Build history of the part. All positions in model axes, mm. A direction names the side the tool comes from. Give positions to 0.01 mm unless a question says otherwise; leave off trailing zeros. Order: outer loops, then holes, each group sorted by start corner. A loop starts at its lowest first (then second) coordinate and runs counter-clockwise, first axis right, second up. Notation, with made-up numbers: (9.5, -12.5) - (57.5, -12.5) arc R14 cw to (57.5, 12.5) - close; hole circle Ø6 at (61.5, 39.25). An arc over 180 degrees is marked (long way). Write each question's results on one line, items separated by ' | '. Start each with the question number.
from build123d import *

# Parameters (mm, degrees)
F0_W     = 10
F0_H     = 10
F1_DEPTH = 40
F3_D     = 2.5
F3_DEPTH = 10
F3_TIP   = 0.7510757738
F5_D     = 2.5
F5_DEPTH = 10
F5_TIP   = 0.7510757738


with BuildPart() as f1:
    # F0 (on Right) → F1 (new body)
    with BuildSketch(Plane.YZ):
        with Locations((-5, 5)):
            Rectangle(F0_W, F0_H)
    extrude(amount=F1_DEPTH)

    # F3
    with Locations(Plane.YZ.offset(40)):
        with Locations((-5, 5)):
            Hole(F3_D / 2, depth=F3_DEPTH)
            with Locations((0, 0, -(F3_DEPTH + F3_TIP / 2))):  # 118° drill point
                Cone(0, F3_D / 2, F3_TIP, mode=Mode.SUBTRACT)

    # F5
    with Locations(Plane(origin=(0, 0, 0), x_dir=(0, -1, 0), z_dir=(-1, 0, 0))):
        with Locations((5, 5)):
            Hole(F5_D / 2, depth=F5_DEPTH)
            with Locations((0, 0, -(F5_DEPTH + F5_TIP / 2))):  # 118° drill point
                Cone(0, F5_D / 2, F5_TIP, mode=Mode.SUBTRACT)


solid = f1.part
Item 1: Which spindle directions (+Z, -Z, +X, -X, +Y, -Y) get a long thin tool onto all of the face, cutting with end or side? Do faces 1 (the cylindrical face through (34.93, -4.73, 3.78)), 2 (the cylindrical face through (5.07, -5.27, 3.78)), 3 (the flat face through (20, -10, 5)). Say none if no direction does.
Item 2: Cut at A-A, the plane x = 35.5. List the corners of the cut face in (y, z), then the cut area to 3 significant figures.
Item 3: Probe line 1 along Y through (x, z) = (35, 5); line 2 along Z through (x, y) = (7.5, -5); line 3 along Z through (x, y) = (6.5, -4.5). List the from-to ranges inside material, lowest first. Write a range as from..to.
Item 4: Two-plate mould, pull along Z, no slides. Class faces 4 (the conical face through (29.38, -5.16, 5.15)), 5 (the conical face through (10.62, -4.84, 5.15)), 6 (the flat face through (20, -5, 0)), 7 (the flat face through (20, 0, 5)): +Z half, -Z half, draft (parallel to the pull), parting line (faces both ways), or undercut.
Item 5: Flat gauge pins, fed straight in: pin 1 Ø1.5 at (y, z) = (-5, 5) entering from +X; pin 2 Ø2 at (y, z) = (-5, 5) entering from +X. Where does each tip first touch, or does it go through?
Values found:
1) face 1: +X | face 2: -X | face 3: +Z, -Z, +X, -X, -Y
2) outline: (-10, 0) - (0, 0) - (0, 10) - (-10, 10) - close; hole circle Ø2.5 at (-5, 5) | area: 95.1 mm2
3) line 1: y = -10..-6.25, -3.75..0 | line 2: z = 0..3.75, 6.25..10 | line 3: z = 0..3.85, 6.15..10
4) face 4: undercut | face 5: undercut | face 6: -Z half | face 7: draft
5) pin 1: stops at x = 29.7 | pin 2: stops at x = 29.85
